from build123d import *

# Parameters (mm, degrees)
HUB_DISC_OD28_THICKNESS4_PROFILE_R            = 14
HUB_DISC_OD28_THICKNESS4_DEPTH                = 4
MG996R_SPLINE_PRESS_SOCKET_D5P80_DEP_2_R      = 2.9
MG996R_SPLINE_PRESS_SOCKET_D5P80_DEPTH3_DEPTH = 3
M3_CENTRE_SCREW_CLEARANCE_THROUGH_FLOOR_START = -50
M3_CENTRE_SCREW_CLEARANCE_THROUGH_FL_2_R      = 1.7
M3_CENTRE_SCREW_CLEARANCE_THROUGH_FLOOR_DEPTH = 71.199009877
LINK_M3_CLEARANCE_PCD18_START                 = -50
LINK_M3_CLEARANCE_PCD18_PROFILE_R             = 1.7
LINK_M3_CLEARANCE_PCD18_DEPTH                 = 71.199009877
CAPTURED_M3_NUT_POCKETS_DEPTH2P9_DEPTH        = 2.9


with BuildPart() as part:
    # Hub_disc_OD28_thickness4_profile → Hub_disc_OD28_thickness4 (new body)
    with BuildSketch(Plane.XY):
        Circle(HUB_DISC_OD28_THICKNESS4_PROFILE_R)
    extrude(amount=HUB_DISC_OD28_THICKNESS4_DEPTH)

    # MG996R_spline_press_socket_D5p80_dep 2 → MG996R_spline_press_socket_D5p80_depth3 (cut)
    with BuildSketch(Plane.XY):
        Circle(MG996R_SPLINE_PRESS_SOCKET_D5P80_DEP_2_R)
    extrude(amount=MG996R_SPLINE_PRESS_SOCKET_D5P80_DEPTH3_DEPTH, mode=Mode.SUBTRACT)

    # M3_centre_screw_clearance_through_fl 2 → M3_centre_screw_clearance_through_floor (cut, through all)
    with BuildSketch(Plane.XY.offset(M3_CENTRE_SCREW_CLEARANCE_THROUGH_FLOOR_START)):
        Circle(M3_CENTRE_SCREW_CLEARANCE_THROUGH_FL_2_R)
    extrude(amount=M3_CENTRE_SCREW_CLEARANCE_THROUGH_FLOOR_DEPTH, mode=Mode.SUBTRACT)

    # Link_M3_clearance_PCD18_profile → Link_M3_clearance_PCD18 (cut, through all)
    with BuildSketch(Plane.XY.offset(LINK_M3_CLEARANCE_PCD18_START)):
        with Locations((9, 0)):
            Circle(LINK_M3_CLEARANCE_PCD18_PROFILE_R)
        with Locations((0, 9)):
            Circle(LINK_M3_CLEARANCE_PCD18_PROFILE_R)
        with Locations((-9, 0)):
            Circle(LINK_M3_CLEARANCE_PCD18_PROFILE_R)
        with Locations((0, -9)):
            Circle(LINK_M3_CLEARANCE_PCD18_PROFILE_R)
    extrude(amount=LINK_M3_CLEARANCE_PCD18_DEPTH, mode=Mode.SUBTRACT)

    # Captured_M3_nut_pockets_AF5p7_profile → Captured_M3_nut_pockets_depth2p9 (cut)
    with BuildSketch(Plane.XY):
        Polygon((11.85, 1.645448267), (9, 3.290896534), (6.15, 1.645448267), (6.15, -1.645448267), (9, -3.290896534), (11.85, -1.645448267), align=None)
        Polygon((-1.645448267, 11.85), (-3.290896534, 9), (-1.645448267, 6.15), (1.645448267, 6.15), (3.290896534, 9), (1.645448267, 11.85), align=None)
        Polygon((-11.85, -1.645448267), (-9, -3.290896534), (-6.15, -1.645448267), (-6.15, 1.645448267), (-9, 3.290896534), (-11.85, 1.645448267), align=None)
        Polygon((1.645448267, -11.85), (3.290896534, -9), (1.645448267, -6.15), (-1.645448267, -6.15), (-3.290896534, -9), (-1.645448267, -11.85), align=None)
    extrude(amount=CAPTURED_M3_NUT_POCKETS_DEPTH2P9_DEPTH, mode=Mode.SUBTRACT)


solid = part.part
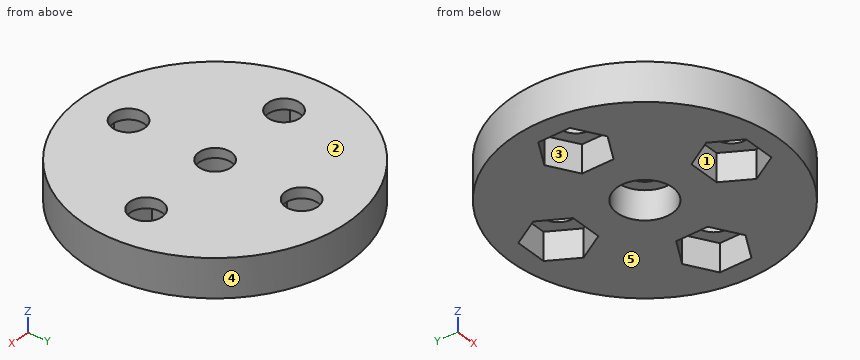
Build history of the part. All positions in model axes, mm. Face numbers are marked on the shaded views. A direction names the side the tool comes from. Give positions to 0.01 mm unless a question says otherwise; leave off trailing zeros. Loops run counter-clockwise (first coordinate to the right, second up) from the corner with the lowest first, then second, coordinate; pieces in that order, holes last. Notation, with made-up numbers: (31, 8.25) - (59, 8.25) arc R22 cw to (59, 25.25) - close; hole circle Ø2 at (51, 53.5). An arc over 180 degrees is marked (long way). Write item = value, one per line. Start each with the question number.
1) Tool access for the marked faces 1 and 2: list every direction of +Z, -Z, +X, -X, +Y, -Y with a clear straight run to the whole face (end or side of a thin tool).
2) Probe probe 1 along Y at (x, z) = (0, 3.4); probe 2 along Y at (x, z) = (0, 2.4); probe 3 along Y at (x, z) = (3, 2.25). List the from-to ranges inside material, lowest first. Write a range as from..to.
3) Band-saw the part on D-D on x = -7.75. Give the cut face in (y, z), plus the area to 3 significant figures.
4) Drop flat-ended pins along their axis: pin 1 Ø3 at (x, y) = (9.5, 0) entering from -Z; pin 2 Ø1.4 at (y, z) = (-0.5, 1.5) entering from +X; pin 3 Ø1.5 at (y, z) = (-4, 1) entering from -X; pin 4 Ø2 at (x, z) = (4.5, 3) entering from +Y. Give the stop position or say it passes through.
5) Band-saw the part on C-C on z = 1. Give the cut face in (x, y), plus the area to 3 significant figures.
6) Pull direction X, two halves, no side cores. Call the marked faces 3, 4 and 5: +X half, -X half, draft (parallel to the pull), parting line (faces both ways), or undercut.
7) Band-saw the part on A-A on y = 0. Give the cut face in (x, z).
Final values:
q1.face_1 = -Z
q1.face_2 = +Z, +X, -X, +Y, -Y
q2.probe_1 = -14..-10.7, -7.3..-1.7, 1.7..7.3, 10.7..14
q2.probe_2 = -14..-11.85, -6.15..-2.9, 2.9..6.15, 11.85..14
q2.probe_3 = -13.67..-9.5, -8.5..8.5, 9.5..13.67
q3.outline = (-11.66, 0) - (-2.57, 0) - (-2.57, 2.9) - (-1.15, 2.9) - (-1.15, 4) - (-11.66, 4) - close; (1.15, 2.9) - (2.57, 2.9) - (2.57, 0) - (11.66, 0) - (11.66, 4) - (1.15, 4) - close
q3.area = 75.8 mm²
q4.pin_1 = 2.9
q4.pin_2 = 14
q4.pin_3 = -13.62
q4.pin_4 = 13.56
q5.outline = circle Ø28 at (0, 0); hole (-11.85, -1.65) - (-9, -3.29) - (-6.15, -1.65) - (-6.15, 1.65) - (-9, 3.29) - (-11.85, 1.65) - close; hole (-3.29, -9) - (-1.65, -11.85) - (1.65, -11.85) - (3.29, -9) - (1.65, -6.15) - (-1.65, -6.15) - close; hole (-3.29, 9) - (-1.65, 6.15) - (1.65, 6.15) - (3.29, 9) - (1.65, 11.85) - (-1.65, 11.85) - close; hole circle Ø5.8 at (0, 0); hole (6.15, -1.65) - (9, -3.29) - (11.85, -1.65) - (11.85, 1.65) - (9, 3.29) - (6.15, 1.65) - close
q5.area = 477 mm²
q6.face_3 = undercut
q6.face_4 = parting line
q6.face_5 = draft
q7.outline = (-14, 0) - (-11.85, 0) - (-11.85, 2.9) - (-10.7, 2.9) - (-10.7, 4) - (-14, 4) - close; (-7.3, 2.9) - (-6.15, 2.9) - (-6.15, 0) - (-2.9, 0) - (-2.9, 3) - (-1.7, 3) - (-1.7, 4) - (-7.3, 4) - close; (1.7, 3) - (2.9, 3) - (2.9, 0) - (6.15, 0) - (6.15, 2.9) - (7.3, 2.9) - (7.3, 4) - (1.7, 4) - close; (10.7, 2.9) - (11.85, 2.9) - (11.85, 0) - (14, 0) - (14, 4) - (10.7, 4) - close
